Work out the finished part from the listing and answer in its coordinate system (mm). Face numbers are marked on the shaded views. A direction names the side the tool comes from. Give positions to 0.01 mm unless a question says otherwise; leave off trailing zeros. Write each loop counter-clockwise with the first axis right and the second up, starting at its lowest first coordinate (ties: lowest second). Pieces come first, ordered by that corner, then holes. Notation, with made-up numbers: (3.5, 53.5) -> (31.5, 53.5) arc R27 ccw to (31.5, 90.5) -> close; hole circle Ø4 at (-1, 55). An arc over 180 degrees is marked (long way). Use a Markdown table: item, result. Add a question column.
Q1. Section B-B, the plane x = -12.5 is taken. Give the vertices of the cut face in (y, z), plus the area to 3 significant figures.
Q2. Each of these flat-tipped pins is pushed along its axis until it touches: pin 1 Ø1 at (y, z) = (11.5, 24) entering from +X; pin 2 Ø1.5 at (x, z) = (-11, 18) entering from -Y. Where does it stop, or does it pass through?
Q3. Consider line 1 (X direction, y = 26, z = 48); line 2 (Y direction, x = -25, z = 32.5); line 3 (Y direction, x = 11.5, z = 54). Determine where each line is inside the solid, lowest interval first.
Q4. Section C-C, the plane z = 32.5 is taken. Give the vertices of the cut face in (x, y).
Q5. Section A-A, the plane z = 39 is taken. Give the vertices of the cut face in (x, y), plus the area to 3 significant figures.
Q6. Section D-D, the plane x = -20 is taken. Give the vertices of the cut face in (y, z).
Q7. For the marked faces 1 and 2, determine the directions among +Z, -Z, +X, -X, +Y, -Y from which every point of the face is accessible in a straight line to the end or side of a thin tool.
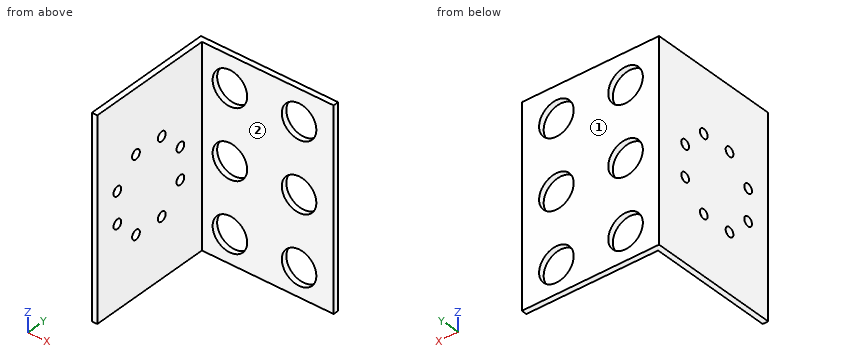
from build123d import *

# Parameters (mm, degrees)
BOSS_EXTRUDE1_DEPTH = 57.15
SKETCH3_R           = 1.35
CUT_EXTRUDE1_DEPTH  = 2.5875
SKETCH2_R           = 5
CUT_EXTRUDE2_DEPTH  = 2.5875


with BuildPart() as part:
    # Sketch1 → Boss-Extrude1 (new body)
    with BuildSketch(Plane.XY):
        Polygon((-25.651653512, -10.718726646), (-24.064153512, -10.718726646), (-24.064153512, 25.793773354), (14.035846488, 25.793773354), (14.035846488, 27.381273354), (-24.064153512, 27.381273354), (-25.651653512, 27.381273354), align=None)
    extrude(amount=BOSS_EXTRUDE1_DEPTH)

    # Sketch3 → Cut-Extrude1 (cut, through all)
    with BuildSketch(Plane(origin=(-24.064153512, 0, 0), x_dir=(0, 0, -1), z_dir=(1, 0, 0))):
        with Locations((-32.5, 18.281273354)):
            Circle(SKETCH3_R)
        with Locations((-23.5, 18.281273354)):
            Circle(SKETCH3_R)
        with Locations((-17, 11.781273354)):
            Circle(SKETCH3_R)
        with Locations((-17, 2.781273354)):
            Circle(SKETCH3_R)
        with Locations((-23.5, -3.718726646)):
            Circle(SKETCH3_R)
        with Locations((-32.5, -3.718726646)):
            Circle(SKETCH3_R)
        with Locations((-39, 2.781273354)):
            Circle(SKETCH3_R)
        with Locations((-39, 11.781273354)):
            Circle(SKETCH3_R)
    extrude(amount=-CUT_EXTRUDE1_DEPTH, mode=Mode.SUBTRACT)

    # Sketch2 → Cut-Extrude2 (cut, through all)
    with BuildSketch(Plane.XZ.offset(-25.793773354)):
        with Locations((4.035846488, 48.15)):
            Circle(SKETCH2_R)
        with Locations((4.035846488, 28.15)):
            Circle(SKETCH2_R)
        with Locations((4.035846488, 8.15)):
            Circle(SKETCH2_R)
        with Locations((-15.964153512, 48.15)):
            Circle(SKETCH2_R)
        with Locations((-15.964153512, 28.15)):
            Circle(SKETCH2_R)
        with Locations((-15.964153512, 8.15)):
            Circle(SKETCH2_R)
    extrude(amount=-CUT_EXTRUDE2_DEPTH, mode=Mode.SUBTRACT)


solid = part.part
Result set:
| question | item | result |
|---|---|---|
| 1 | outline | (25.79, 0) -> (27.38, 0) -> (27.38, 4.54) -> (25.79, 4.54) -> close; (25.79, 11.76) -> (27.38, 11.76) -> (27.38, 24.54) -> (25.79, 24.54) -> close; (25.79, 31.76) -> (27.38, 31.76) -> (27.38, 44.54) -> (25.79, 44.54) -> close; (25.79, 51.76) -> (27.38, 51.76) -> (27.38, 57.15) -> (25.79, 57.15) -> close |
| 1 | area | 56.4 mm2 |
| 2 | pin 1 | stops at x = -24.06 |
| 2 | pin 2 | stops at y = 25.79 |
| 3 | line 1 | x = -25.65 to -20.96, -10.97 to -0.96, 9.03 to 14.04 |
| 3 | line 2 | y = -10.72 to -5.07, -2.37 to 16.93, 19.63 to 27.38 |
| 3 | line 3 | y = 25.79 to 27.38 |
| 4 | outline | (-25.65, -10.72) -> (-24.06, -10.72) -> (-24.06, -5.07) -> (-25.65, -5.07) -> close; (-25.65, -2.37) -> (-24.06, -2.37) -> (-24.06, 16.93) -> (-25.65, 16.93) -> close; (-25.65, 19.63) -> (-24.06, 19.63) -> (-24.06, 25.79) -> (-18.43, 25.79) -> (-18.43, 27.38) -> (-25.65, 27.38) -> close; (-13.5, 25.79) -> (1.57, 25.79) -> (1.57, 27.38) -> (-13.5, 27.38) -> close; (6.5, 25.79) -> (14.04, 25.79) -> (14.04, 27.38) -> (6.5, 27.38) -> close |
| 5 | outline | (-25.65, -10.72) -> (-24.06, -10.72) -> (-24.06, 1.43) -> (-25.65, 1.43) -> close; (-25.65, 4.13) -> (-24.06, 4.13) -> (-24.06, 10.43) -> (-25.65, 10.43) -> close; (-25.65, 13.13) -> (-24.06, 13.13) -> (-24.06, 25.79) -> (14.04, 25.79) -> (14.04, 27.38) -> (-25.65, 27.38) -> close |
| 5 | area | 112 mm2 |
| 6 | outline | (25.79, 0) -> (27.38, 0) -> (27.38, 5.2) -> (25.79, 5.2) -> close; (25.79, 11.1) -> (27.38, 11.1) -> (27.38, 25.2) -> (25.79, 25.2) -> close; (25.79, 31.1) -> (27.38, 31.1) -> (27.38, 45.2) -> (25.79, 45.2) -> close; (25.79, 51.1) -> (27.38, 51.1) -> (27.38, 57.15) -> (25.79, 57.15) -> close |
| 7 | face 1 | +Z, -Z, +X, -X, +Y |
| 7 | face 2 | +Z, -Z, +X, -Y |
